For this review, take the finished solid that the model builds, in its own axes (mm). Round coordinates to 2 decimals unless told otherwise and drop trailing zeros. Write each loop counter-clockwise with the first axis right and the second up, starting at its lowest first coordinate (ties: lowest second). Pieces come first, ordered by that corner, then holes. Notation, with made-up numbers: (-27, 78.25) - (15, 78.25) arc R31 ccw to (15, 117.25) - close; hole circle Ø3 at (73, -29). An arc over 180 degrees is marked (long way). One line per item, written item: value. Start each with the question number.
Q1. Add section A-A on z = 13.4. Write out the cut boundary in (x, y), and give its area (3 significant figures).
Q2. Clearance check with flat-ended pins moving along their axes: pin 1 Ø4 at (x, z) = (6.8, 96.4) entering from +Y; pin 2 Ø7 at (x, z) = (217.8, 96.4) entering from +Y. State where each tip first meets the part, or that it passes through.
Q3. Mouldability with a two-part tool opening along Z and no side actions: class faces 1 (the face through (223, 1.5, 2.1)), 2 (the face through (2, 1.5, 107.9)), 3 (the face through (6.51, 1.52, 15.63)) as +Z half, -Z half, draft (parallel to the pull), parting line (faces both ways), or undercut.
Q4. For probe 1 along Z at (x, y) = (6.8, 0.9); probe 2 along X at (y, z) = (2.45, 103.5); probe 3 along X at (y, z) = (2, 15), list the stretches that pass through material, from the lowest coordinate up.
```python
from build123d import *

# Parameters (mm, degrees)
CYLINDER007_R     = 2.25
CYLINDER007_DEPTH = 3
CYLINDER006_R     = 2.25
CYLINDER006_DEPTH = 3
CYLINDER005_R     = 2.25
CYLINDER005_DEPTH = 3
CYLINDER_R        = 2.25
CYLINDER_DEPTH    = 3
BOX_W             = 225
BOX_H             = 3
BOX_DEPTH         = 110
FILLET_R          = 7


with BuildPart() as cylinder007:
    # Cylinder007 → Cylinder007 (new body)
    with BuildSketch(Plane(origin=(217.8, -18, 13.4), x_dir=(1, 0, 0), z_dir=(0, -1, 0))):
        Circle(CYLINDER007_R)
    extrude(amount=CYLINDER007_DEPTH)


with BuildPart() as fusion005:
    # Cylinder006 → Cylinder006 (new body)
    with BuildSketch(Plane(origin=(217.8, -18, 96.4), x_dir=(1, 0, 0), z_dir=(0, -1, 0))):
        Circle(CYLINDER006_R)
    extrude(amount=CYLINDER006_DEPTH)

    # Fusion005: union Cylinder007
    add(cylinder007.part)


with BuildPart() as cylinder005:
    # Cylinder005 → Cylinder005 (new body)
    with BuildSketch(Plane(origin=(6.8, -18, 96.4), x_dir=(1, 0, 0), z_dir=(0, -1, 0))):
        Circle(CYLINDER005_R)
    extrude(amount=CYLINDER005_DEPTH)


with BuildPart() as screw_holes:
    # Cylinder → Cylinder (new body)
    with BuildSketch(Plane(origin=(6.8, -18, 13.4), x_dir=(1, 0, 0), z_dir=(0, -1, 0))):
        Circle(CYLINDER_R)
    extrude(amount=CYLINDER_DEPTH)

    # Fusion004: union Cylinder005
    add(cylinder005.part)

    # Fusion006: union Fusion005
    add(fusion005.part)


with BuildPart() as screw_holes_1:
    # Fusion006 placement: moved
    add(screw_holes.part.moved(Location((0, 21, 0))))


with BuildPart() as cut009:
    # Box → Box (new body)
    with BuildSketch(Plane.XY):
        with Locations((112.5, 1.5)):
            Rectangle(BOX_W, BOX_H)
    extrude(amount=BOX_DEPTH)

    # Fillet
    fillet_edges = [cut009.edges().sort_by_distance(p)[0] for p in [
        (0, 1.5, 110),
        (0, 1.5, 0),
        (225, 1.5, 110),
        (225, 1.5, 0),
    ]]
    fillet(fillet_edges, radius=FILLET_R)

    # Cut009: cut Screw Holes
    add(screw_holes_1.part, mode=Mode.SUBTRACT)


solid = cut009.part
```
Result set:
1. outline: (0, 0) - (4.55, 0) - (4.55, 3) - (0, 3) - close; (9.05, 0) - (215.55, 0) - (215.55, 3) - (9.05, 3) - close; (220.05, 0) - (225, 0) - (225, 3) - (220.05, 3) - close
1. area: 648 mm^2
2. pin 1: passes through
2. pin 2: stops at y = 3
3. face 1: -Z half
3. face 2: +Z half
3. face 3: undercut
4. probe 1: z = 0 to 11.15, 15.65 to 94.15, 98.65 to 110
4. probe 2: x = 0.02 to 224.98
4. probe 3: x = 0 to 5.22, 8.38 to 216.22, 219.38 to 225
